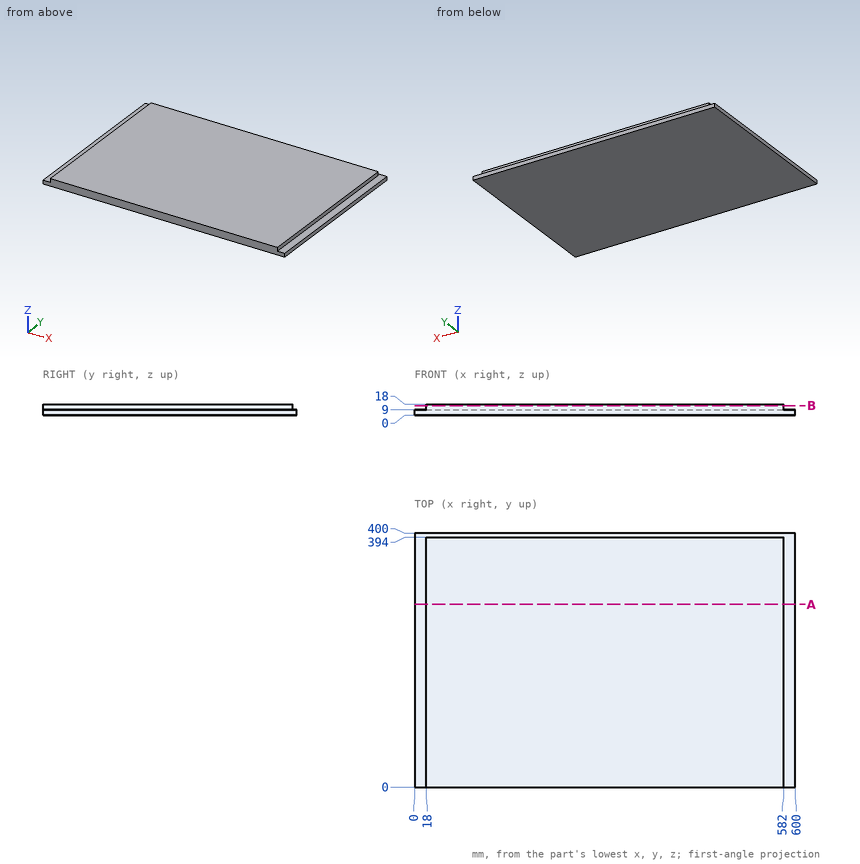
Design review of the part shown in the three views and the two pictorial views. Dimensions are in mm from the part's minimum x, y and z. Round coordinates to 2 decimals unless told otherwise and drop trailing zeros. Write each loop counter-clockwise with the first axis right and the second up, starting at its lowest first coordinate (ties: lowest second). Pieces come first, ordered by that corner, then holes. Notation, with made-up numbers: M -22.75,42 L 27.25,42 A6 cw 27.25,49 Z; hole C 19.25,22.25 d8. An arc over 180 degrees is marked long. Use a Markdown table: item, result. Add a question column.
Q1. We need section B-B, the plane z = 15.25. State the section outline as (x, y) points, plus the area to 3 significant figures.
Q2. To check wall thickness, follow line 1 (Y direction, x = 221, z = 13.5); line 2 (X direction, y = 373, z = 14.75). State the ranges of each line that lie inside material, in increasing order.
Q3. Insertion check: pin 1 (3 mm diameter, centred on y = 322, z = 12, fed in from +X); pin 2 (2.5 mm diameter, centred on y = 190, z = 13.5, fed in from -X). Each pin has a flat end and moves straight along its axis. Give the tip position at first contact, or say it passes through.
Q4. We need section A-A, the plane y = 288. State the section outline as (x, z) points, plus the area to 3 significant figures.
Findings below:
| question | item | result |
|---|---|---|
| 1 | outline | M 18,0 L 582,0 L 582,394 L 18,394 Z |
| 1 | area | 222,000 mm² |
| 2 | line 1 | y = 0 to 394 |
| 2 | line 2 | x = 18 to 582 |
| 3 | pin 1 | stops at x = 582 |
| 3 | pin 2 | stops at x = 18 |
| 4 | outline | M 0,0 L 600,0 L 600,9 L 582,9 L 582,18 L 18,18 L 18,9 L 0,9 Z |
| 4 | area | 10,500 mm² |
